Source: CAD feature listing. Evaluate the final solid. Frame: model axes, mm. A direction names the side the tool comes from. Round coordinates to 2 decimals unless told otherwise and drop trailing zeros. Write each loop counter-clockwise with the first axis right and the second up, starting at its lowest first coordinate (ties: lowest second). Pieces come first, ordered by that corner, then holes.
from build123d import *

# Parameters (mm, degrees)
Y_KSEKLIK_EKSTR_ZYON1_DEPTH = 9.3
KES_EKSTR_ZYON1_DEPTH       = 10.3
KES_EKSTR_ZYON2_DEPTH       = 37
IZIM4_W                     = 4
IZIM4_H                     = 7
KES_EKSTR_ZYON3_DEPTH       = 25


with BuildPart() as part:
    # Çizim1 → Yükseklik-Ekstrüzyon1 (new body)
    with BuildSketch(Plane(origin=(0, 0, 0), x_dir=(1, 0, 0), z_dir=(0, 1, 0))):
        with BuildLine():
            Line((18, -11.757976016), (18, 11.757976016))
            ThreePointArc((18, 11.757976016), (0, 21.5), (-18, 11.757976016))
            Line((-18, 11.757976016), (-18, -11.757976016))
            ThreePointArc((-18, -11.757976016), (0, -21.5), (18, -11.757976016))
        make_face()
    extrude(amount=-Y_KSEKLIK_EKSTR_ZYON1_DEPTH)

    # Çizim2 → Kes-Ekstrüzyon1 (cut, through all)
    with BuildSketch(Plane(origin=(0, 0, 0), x_dir=(1, 0, 0), z_dir=(0, 1, 0))):
        with BuildLine():
            Line((8.25, -14.75), (15.642490211, -14.75))
            ThreePointArc((15.642490211, -14.75), (12.215804254, -17.692487853), (8.25, -19.854155736))
            Line((8.25, -19.854155736), (8.25, -14.75))
        make_face()
        with BuildLine():
            Line((-8.25, -19.854155736), (-8.25, -14.75))
            Line((-8.25, -14.75), (-15.642490211, -14.75))
            ThreePointArc((-15.642490211, -14.75), (-12.215804254, -17.692487853), (-8.25, -19.854155736))
        make_face()
        with BuildLine():
            Line((8.25, 14.75), (15.642490211, 14.75))
            ThreePointArc((15.642490211, 14.75), (12.215804254, 17.692487853), (8.25, 19.854155736))
            Line((8.25, 19.854155736), (8.25, 14.75))
        make_face()
        with BuildLine():
            Line((-15.642490211, 14.75), (-8.25, 14.75))
            Line((-8.25, 14.75), (-8.25, 19.854155736))
            ThreePointArc((-8.25, 19.854155736), (-12.215804254, 17.692487853), (-15.642490211, 14.75))
        make_face()
    extrude(amount=-KES_EKSTR_ZYON1_DEPTH, mode=Mode.SUBTRACT)

    # Çizim3 → Kes-Ekstrüzyon2 (cut, through all)
    with BuildSketch(Plane(origin=(18, 0, 0), x_dir=(0, 0, -1), z_dir=(1, 0, 0))):
        with BuildLine():
            Line((-7.25, -2.25), (-7.25, 1))
            Line((-7.25, 1), (-12.75, 1))
            Line((-12.75, 1), (-12.75, -2.25))
            ThreePointArc((-12.75, -2.25), (-10, -5), (-7.25, -2.25))
        make_face()
        with BuildLine():
            Line((12.75, -2.25), (12.75, 1))
            Line((12.75, 1), (7.25, 1))
            Line((7.25, 1), (7.25, -2.25))
            ThreePointArc((7.25, -2.25), (10, -5), (12.75, -2.25))
        make_face()
    extrude(amount=-KES_EKSTR_ZYON2_DEPTH, mode=Mode.SUBTRACT)

    # Çizim4 → Kes-Ekstrüzyon3 (cut, symmetric)
    with BuildSketch(Plane.XY):
        with Locations((-10.25, -3.5)):
            Rectangle(IZIM4_W, IZIM4_H)
        with Locations((10.25, -3.5)):
            Rectangle(IZIM4_W, IZIM4_H)
    extrude(amount=KES_EKSTR_ZYON3_DEPTH, both=True, mode=Mode.SUBTRACT)


solid = part.part
1) Section query B-B on z = -10. Return the cut outline in (x, y), then the cut area to 3 significant figures.
Taken from the geometry:
outline: (-18, -9.3) - (18, -9.3) - (18, -5) - (12.25, -5) - (12.25, -7) - (8.25, -7) - (8.25, -5) - (-8.25, -5) - (-8.25, -7) - (-12.25, -7) - (-12.25, -5) - (-18, -5) - close
area: 139 mm2
2) Reachability of faces 1 (the face through (10, -7, 0)), 2 (the face through (-14, -6, -14.75)), 3 (the face through (0, -1, -7.25)), 4 (the face through (14, -6, 14.75)), 5 (the face through (14, -6, -14.75)) from +Z, -Z, +X, -X, +Y, -Y: full face, straight path, thin tool, end or side. Return the list, or none.
Taken from the geometry:
face 1: +Z, -Z, +Y
face 2: -Z, -X, +Y, -Y
face 3: +X, -X, +Y
face 4: +Z, +X, +Y, -Y
face 5: -Z, +X, +Y, -Y
3) Pull-direction query (Z, two-part tool) for faces 6 (the face through (0, -1, 7.25)), 7 (the face through (-0.1, -4.6, 21.5)), 8 (the face through (-18, -6, 0)); classes: released by +Z, released by -Z, zero draft, split by the parting line, or undercut.
Taken from the geometry:
face 6: undercut
face 7: released by +Z
face 8: zero draft
4) Contact query for flat-ended pins moving along their axis: P1, Ø2.5, axis at x = 0.5, y = -1.5, coming from the -Z side; P2, Ø0.7, axis at x = 14.5, y = -0.5, coming from the -Z side; P3, Ø1.8, axis at x = -14.5, y = -1, coming from the +Z side. Output: stop coordinate, or through.
Taken from the geometry:
P1: stops at z = -21.5
P2: stops at z = -14.75
P3: stops at z = 14.75
5) Material intervals for line 1 (X direction, y = -4.75, z = 5.5); line 2 (Z direction, x = 14.5, y = -3.75); line 3 (Z direction, x = 3, y = -2.75), sorted ascending.
Taken from the geometry:
line 1: x = -18 to -12.25, -8.25 to 8.25, 12.25 to 18
line 2: z = -14.75 to -12.3, -7.7 to 7.7, 12.3 to 14.75
line 3: z = -21.29 to -12.7, -7.3 to 7.3, 12.7 to 21.29
6) Section query C-C on x = 6.5. Return the cut outline in (y, z).
Taken from the geometry:
outline: (-9.3, -20.49) - (0, -20.49) - (0, -12.75) - (-2.25, -12.75) arc R2.75 cw to (-2.25, -7.25) - (0, -7.25) - (0, 7.25) - (-2.25, 7.25) arc R2.75 cw to (-2.25, 12.75) - (0, 12.75) - (0, 20.49) - (-9.3, 20.49) - close
7) Section query A-A on y = -6.5. Return the cut outline in (x, z), then the cut area to 3 significant figures.
Taken from the geometry:
outline: (-18, -11.76) arc R21.5 ccw to (-15.64, -14.75) - (-12.25, -14.75) - (-12.25, 14.75) - (-15.64, 14.75) arc R21.5 ccw to (-18, 11.76) - close; (-8.25, -19.85) arc R21.5 ccw to (8.25, -19.85) - (8.25, 19.85) arc R21.5 ccw to (-8.25, 19.85) - close; (12.25, -14.75) - (15.64, -14.75) arc R21.5 ccw to (18, -11.76) - (18, 11.76) arc R21.5 ccw to (15.64, 14.75) - (12.25, 14.75) - close
area: 1,020 mm2
8) Section query D-D on y = -0.75. State how many separate pieces and enclosed holes the cut face has, then the cut area to 3 significant figures.
Taken from the geometry:
separate pieces: 9
enclosed holes: 0
area: 711 mm2
